Read the model definition and answer for the solid it produces. Units are mm, in the model's axes. A direction names the side the tool comes from. Coordinates: 2 decimals unless noted, no trailing zeros. Write each loop counter-clockwise with the first axis right and the second up, starting at its lowest first coordinate (ties: lowest second). Pieces come first, ordered by that corner, then holes.
Item 1: Straight lines are drawn through the part: probe 1 along Y at (x, z) = (0, 7.5) (3 decimals); probe 2 along Z at (x, y) = (3.5, -5.25); probe 3 along X at (y, z) = (0.75, 11). For each, find the intervals that lie inside material, in ascending order.
Item 2: Each of these flat-tipped pins is pushed along its axis until it touches: P1, Ø4, axis at x = -3, y = -1.5, coming from the +Z side; P2, Ø1.9, axis at x = 0, y = 0.5, coming from the -Z side; P3, Ø1, axis at y = -3.5, z = 59, coming from the -X side. Where does it stop, or does it pass through?
Item 3: Determine the mould class of faces 1 (the face through (0, 0, 12.7)), 2 (the face through (1, -2, 0)), 3 (the face through (3.997, 1.259, 36.314)) for opening direction Y: released by +Y, released by -Y, zero draft, split by the parting line, or undercut.
Item 4: Section A-A (z = 14) is taken. Give the vertices of the cut face in (x, y), then the cut area to 3 significant figures.
Item 5: Section C-C (x = 5.5) is taken. Give the vertices of the cut face in (y, z).
Item 6: A tool of negligible diameter and unlimited length cuts with its end or side. For faces 4 (the face through (1.32, -4.14, 73.66)), 5 (the face through (-1.38, -6.2, 74.29)), 6 (the face through (3, 2, 74.93)), from which of +Z, -Z, +X, -X, +Y, -Y can it reach the whole face along a straight path? Write none if from no direction.
Item 7: Section B-B (y = -5.25) is taken. Give the vertices of the cut face in (x, z).
from build123d import *

# Parameters (mm, degrees)
F0_R     = 4.191
F1_DEPTH = 73.66
F2_R     = 4.191
F3_DEPTH = 8.382
F4_R     = 4.19099
F5_R     = 6.35
F6_DEPTH = 1.27
F7_R     = 1.905
F8_DEPTH = 12.7


# Not quite as in the source:
# - a fillet or chamfer is up to 0.001 mm smaller than in the source, because OpenCascade refuses the exact size


with BuildPart() as f1:
    # F0 (on Top) → F1 (new body)
    with BuildSketch(Plane.XY):
        Circle(F0_R)
    extrude(amount=F1_DEPTH)



with BuildPart() as f3:
    # F2 (on face) → F3 (new body)
    with BuildSketch(Plane.XY.offset(73.66)):
        Circle(F2_R)
    extrude(amount=F3_DEPTH)

    # F4 (radius 4.191 in the source; OpenCascade refuses exactly that, so slightly less here)
    f4_edges = [f3.edges().sort_by_distance(p)[0] for p in [
        (-4.191, 0, 73.66),
        (-4.191, 0, 82.042),
    ]]
    fillet(f4_edges, radius=F4_R)


with BuildPart() as f1_1:
    add(f1.part)

    add(f3.part)  # F6 merges F3
    # F5 (on face) → F6 (join)
    with BuildSketch(Plane.XY.offset(73.66)):
        Circle(F5_R)
    extrude(amount=F6_DEPTH)

    # F7 (on face) → F8 (cut)
    with BuildSketch(Plane(origin=(0, 0, 0), x_dir=(1, 0, 0), z_dir=(0, 0, -1))):
        Circle(F7_R)
    extrude(amount=-F8_DEPTH, mode=Mode.SUBTRACT)


solid = f1_1.part
Established:
1. probe 1: y = -4.191 to -1.905, 1.905 to 4.191
1. probe 2: z = 73.66 to 74.93
1. probe 3: x = -4.12 to -1.75, 1.75 to 4.12
2. P1: stops at z = 81.82
2. P2: stops at z = 12.7
2. P3: stops at x = -2.93
3. face 1: undercut
3. face 2: zero draft
3. face 3: split by the parting line
4. outline: circle Ø8.38 at (0, 0)
4. area: 55.2 mm2
5. outline: (-3.17, 73.66) - (3.17, 73.66) - (3.17, 74.93) - (-3.17, 74.93) - close
6. face 4: -Z
6. face 5: +Z, -Z
6. face 6: none
7. outline: (-3.57, 73.66) - (3.57, 73.66) - (3.57, 74.93) - (-3.57, 74.93) - close
